Design review of the part built by this model. Coordinates are the model's own, in mm. A direction names the side the tool comes from. Coordinates: 2 decimals unless noted, no trailing zeros. Loops run counter-clockwise (first coordinate to the right, second up) from the corner with the lowest first, then second, coordinate; pieces in that order, holes last. Notation, with made-up numbers: (-15, -39.75) -> (26, -39.75) arc R38 ccw to (26, -1.75) -> close; hole circle Ø10 at (-28, -24). An arc over 180 degrees is marked (long way). Answer in a Markdown table with one row per item.
```python
from build123d import *

# Parameters (mm, degrees)
SKETCH_1_W      = 26
SKETCH_1_H      = 30
EXTRUDE_1_DEPTH = 15
SKETCH_2_W      = 46
SKETCH_2_H      = 30
EXTRUDE_2_DEPTH = 2
SKETCH_4_W      = 26
SKETCH_4_H      = 8
EXTRUDE_3_DEPTH = 4


with BuildPart() as part:
    # 草图1 → 凸台-拉伸1 (new body)
    with BuildSketch(Plane.XY):
        with Locations((-460, 0)):
            Rectangle(SKETCH_1_W, SKETCH_1_H)
    extrude(amount=EXTRUDE_1_DEPTH)

    # 草图2 → 凸台-拉伸2 (add)
    with BuildSketch(Plane.XY.offset(15)):
        with Locations((-460, 0)):
            Rectangle(SKETCH_2_W, SKETCH_2_H)
    extrude(amount=EXTRUDE_2_DEPTH)

    # 草图4 → 凸台-拉伸3 (add)
    with BuildSketch(Plane(origin=(0, 0, 0), x_dir=(-1, 0, 0), z_dir=(0, 0, -1))):
        with Locations((460, 0)):
            Rectangle(SKETCH_4_W, SKETCH_4_H)
    extrude(amount=EXTRUDE_3_DEPTH)


solid = part.part
```
(1) Take a section at A-A on y = -0.25. Give the boundary of the cut face in (x, z).
Evaluation:
| item | result |
|---|---|
| outline | (-483, 15) -> (-473, 15) -> (-473, -4) -> (-447, -4) -> (-447, 15) -> (-437, 15) -> (-437, 17) -> (-483, 17) -> close |
(2) Take a section at C-C on z = -2.5. Give the boundary of the cut face in (x, y), and give its area (3 significant figures).
Evaluation:
| item | result |
|---|---|
| outline | (-473, -4) -> (-447, -4) -> (-447, 4) -> (-473, 4) -> close |
| area | 208 mm² |
(3) To check wall thickness, follow probe 1 along X at (y, z) = (-12.75, 10); probe 2 along Z at (x, y) = (-457, -5); probe 3 along Z at (x, y) = (-445, 13.75). State the ranges of each line that lie inside material, in increasing order.
Evaluation:
| item | result |
|---|---|
| probe 1 | x = -473 to -447 |
| probe 2 | z = 0 to 17 |
| probe 3 | z = 15 to 17 |
(4) Take a section at B-B on x = -459.5. Give the boundary of the cut face in (y, z), and give its area (3 significant figures).
Evaluation:
| item | result |
|---|---|
| outline | (-15, 0) -> (-4, 0) -> (-4, -4) -> (4, -4) -> (4, 0) -> (15, 0) -> (15, 17) -> (-15, 17) -> close |
| area | 542 mm² |
(5) Tool access review of faces 1 (the flat face through (-460, -9, 0)), 2 (the flat face through (-478, 0, 15)), 3 (the flat face through (-460, 10, 0)): name each direction out of +Z, -Z, +X, -X, +Y, -Y from which nothing blocks a thin tool from reaching the whole face with its end or side.
Evaluation:
| item | result |
|---|---|
| face 1 | -Z, +X, -X, -Y |
| face 2 | -Z, -X, +Y, -Y |
| face 3 | -Z, +X, -X, +Y |
(6) For pin 1 (8 mm diameter, centred on x = -480.5, y = -5.5, fed in from -Z); pin 2 (5.5 mm diameter, centred on x = -461.5, y = -7, fed in from -Z); pin 3 (5.5 mm diameter, centred on y = 4.5, z = 8.5, fed in from -X); pin 4 (4 mm diameter, centred on x = -463.5, z = -1, fed in from -Y), all flat-tipped, find the tip position at first contact; note any pin that passes through.
Evaluation:
| item | result |
|---|---|
| pin 1 | stops at z = 15 |
| pin 2 | stops at z = 0 |
| pin 3 | stops at x = -473 |
| pin 4 | stops at y = -15 |
(7) Take a section at D-D on x = -475. Give the boundary of the cut face in (y, z).
Evaluation:
| item | result |
|---|---|
| outline | (-15, 15) -> (15, 15) -> (15, 17) -> (-15, 17) -> close |
